```python
from build123d import *

# Parameters (mm, degrees)
SKETCH_1_R                         = 2.25
SM_BASE_FLANGE_1_DEPTH             = 5
FILLET_1_R                         = 30
SM_EDGE_FLANGE_1_STRIP_W           = 28
SM_EDGE_FLANGE_1_STRIP_H           = 5
SM_EDGE_FLANGE_1_STRIP_CUT_DEPTH   = 675
SM_EDGE_FLANGE_1_STRIP_2_W         = 28
SM_EDGE_FLANGE_1_STRIP_2_H         = 5
SM_EDGE_FLANGE_1_STRIP_CUT_2_DEPTH = 675
SM_EDGE_FLANGE_1_DEPTH             = 675
SM_EDGE_FLANGE_1_BEND_DEPTH        = 675
CUT_EXTRUDE_3_REACH                = 892.463
FILLET_2_R                         = 10
SKETCH_12_R                        = 5
CUT_EXTRUDE_4_DEPTH                = 891.463362525


# Sheet-metal steps are written as plain solids
with BuildPart() as part:
    # Sketch 1 → 基体-法兰1 (new body)
    with BuildSketch(Plane.XY):
        Polygon((0, 0), (0, 675), (45, 675), (45, 480), (165, 480), (165, 290), (535, 290), (535, 675), (580, 675), (580, 0), (523, 0), (523, 90), (57, 90), (57, 0), align=None)
        with Locations((154, 458)):
            Circle(SKETCH_1_R, mode=Mode.SUBTRACT)
        with Locations((45, 458)):
            Circle(SKETCH_1_R, mode=Mode.SUBTRACT)
        with Locations((154, 301)):
            Circle(SKETCH_1_R, mode=Mode.SUBTRACT)
        with Locations((45, 301)):
            Circle(SKETCH_1_R, mode=Mode.SUBTRACT)
        with BuildLine():
            Line((80, 133), (110, 133))
            ThreePointArc((110, 133), (150, 173), (110, 213))
            Line((110, 213), (80, 213))
            ThreePointArc((80, 213), (40, 173), (80, 133))
        make_face(mode=Mode.SUBTRACT)
    extrude(amount=-SM_BASE_FLANGE_1_DEPTH)

    # 圆角1
    fillet_1_edges = [part.edges().sort_by_distance(p)[0] for p in [
        (45, 480, -2.5),
        (165, 480, -2.5),
        (165, 290, -2.5),
        (535, 290, -2.5),
        (523, 90, -2.5),
        (57, 90, -2.5),
    ]]
    fillet(fillet_1_edges, radius=FILLET_1_R)

    # 边线-法兰1 strip (across the edge) → 边线-法兰1 strip cut (cut)
    with BuildSketch(Plane.XZ.offset(-675)):
        with Locations((-5, -2.5)):
            Rectangle(SM_EDGE_FLANGE_1_STRIP_W, SM_EDGE_FLANGE_1_STRIP_H)
    extrude(amount=SM_EDGE_FLANGE_1_STRIP_CUT_DEPTH, mode=Mode.SUBTRACT)

    # 边线-法兰1 strip 2 (across the edge) → 边线-法兰1 strip cut 2 (cut)
    with BuildSketch(Plane(origin=(580, 0, 0), x_dir=(-1, 0, 0), z_dir=(0, 1, 0))):
        with Locations((-5, -2.5)):
            Rectangle(SM_EDGE_FLANGE_1_STRIP_2_W, SM_EDGE_FLANGE_1_STRIP_2_H)
    extrude(amount=SM_EDGE_FLANGE_1_STRIP_CUT_2_DEPTH, mode=Mode.SUBTRACT)

    # 边线-法兰1 section (across the edge) → 边线-法兰1 (add)
    with BuildSketch(Plane.XZ.offset(-675)):
        with BuildLine():
            Line((0, 4), (0, 30))
            Line((0, 30), (5, 30))
            Line((5, 30), (5, 4))
            ThreePointArc((5, 4), (6.171572875, 1.171572875), (9, 0))
            Line((9, 0), (9, -5))
            ThreePointArc((9, -5), (2.636038969, -2.363961031), (0, 4))
        make_face()
    extrude(amount=SM_EDGE_FLANGE_1_DEPTH)

    # 边线-法兰1 section 2 (across the edge) → 边线-法兰1 bend (add)
    with BuildSketch(Plane(origin=(580, 0, 0), x_dir=(-1, 0, 0), z_dir=(0, 1, 0))):
        with BuildLine():
            Line((0, 4), (0, 30))
            Line((0, 30), (5, 30))
            Line((5, 30), (5, 4))
            ThreePointArc((5, 4), (6.171572875, 1.171572875), (9, 0))
            Line((9, 0), (9, -5))
            ThreePointArc((9, -5), (2.636038969, -2.363961031), (0, 4))
        make_face()
    extrude(amount=SM_EDGE_FLANGE_1_BEND_DEPTH)

    # 草图11 → 切除-拉伸3 (cut, up to next)
    with BuildSketch(Plane.XY, mode=Mode.PRIVATE) as cut_extrude_3_sk1:
        with BuildLine():
            Line((252.5, 110), (247.5, 110))
            ThreePointArc((247.5, 110), (241.5, 116), (247.5, 122))
            Line((247.5, 122), (252.5, 122))
            ThreePointArc((252.5, 122), (258.5, 116), (252.5, 110))
        make_face()
    cut_extrude_3_tool1 = extrude(cut_extrude_3_sk1.sketch, amount=-CUT_EXTRUDE_3_REACH, mode=Mode.PRIVATE) & part.part
    # 草图11 → 切除-拉伸3 (cut, up to next)
    with BuildSketch(Plane.XY, mode=Mode.PRIVATE) as cut_extrude_3_sk2:
        with BuildLine():
            Line((510.5, 110), (505.5, 110))
            ThreePointArc((505.5, 110), (499.5, 116), (505.5, 122))
            Line((505.5, 122), (510.5, 122))
            ThreePointArc((510.5, 122), (516.5, 116), (510.5, 110))
        make_face()
    cut_extrude_3_tool2 = extrude(cut_extrude_3_sk2.sketch, amount=-CUT_EXTRUDE_3_REACH, mode=Mode.PRIVATE) & part.part
    # 草图11 → 切除-拉伸3 (cut, up to next)
    with BuildSketch(Plane.XY, mode=Mode.PRIVATE) as cut_extrude_3_sk3:
        with BuildLine():
            Line((510.5, 224), (505.5, 224))
            ThreePointArc((505.5, 224), (499.5, 230), (505.5, 236))
            Line((505.5, 236), (510.5, 236))
            ThreePointArc((510.5, 236), (516.5, 230), (510.5, 224))
        make_face()
    cut_extrude_3_tool3 = extrude(cut_extrude_3_sk3.sketch, amount=-CUT_EXTRUDE_3_REACH, mode=Mode.PRIVATE) & part.part
    # 草图11 → 切除-拉伸3 (cut, up to next)
    with BuildSketch(Plane.XY, mode=Mode.PRIVATE) as cut_extrude_3_sk4:
        with BuildLine():
            Line((252.5, 224), (247.5, 224))
            ThreePointArc((247.5, 224), (241.5, 230), (247.5, 236))
            Line((247.5, 236), (252.5, 236))
            ThreePointArc((252.5, 236), (258.5, 230), (252.5, 224))
        make_face()
    cut_extrude_3_tool4 = extrude(cut_extrude_3_sk4.sketch, amount=-CUT_EXTRUDE_3_REACH, mode=Mode.PRIVATE) & part.part
    add(cut_extrude_3_tool1.solids().sort_by_distance((250, 116, 0))[0], mode=Mode.SUBTRACT)
    add(cut_extrude_3_tool2.solids().sort_by_distance((508, 116, 0))[0], mode=Mode.SUBTRACT)
    add(cut_extrude_3_tool3.solids().sort_by_distance((508, 230, 0))[0], mode=Mode.SUBTRACT)
    add(cut_extrude_3_tool4.solids().sort_by_distance((250, 230, 0))[0], mode=Mode.SUBTRACT)

    # 圆角2
    fillet_2_edges = [part.edges().sort_by_distance(p)[0] for p in [
        (2.5, 675, 30),
        (2.5, 0, 30),
        (577.5, 0, 30),
        (577.5, 675, 30),
    ]]
    fillet(fillet_2_edges, radius=FILLET_2_R)

    # 草图12 → 切除-拉伸4 (cut, through all)
    with BuildSketch(Plane(origin=(580, 0, 0), x_dir=(0, 0, -1), z_dir=(1, 0, 0))):
        with Locations((-15, 29)):
            Circle(SKETCH_12_R)
    extrude(amount=-CUT_EXTRUDE_4_DEPTH, mode=Mode.SUBTRACT)


solid = part.part
```
Model file for the job. Use its own axes, mm. A direction names the side the tool comes from. Coordinates: 2 decimals unless noted, no trailing zeros. Write each loop counter-clockwise with the first axis right and the second up, starting at its lowest first coordinate (ties: lowest second). Pieces come first, ordered by that corner, then holes. Notation, with made-up numbers: (41, 52) - (74, 52) arc R5 cw to (74, 58) - close; hole circle Ø2 at (28, -15.5). An arc over 180 degrees is marked (long way). One line per item, written item: value. Start each with the question number.
1. Probe line 1 (X direction, y = 275, z = 24); line 2 (Y direction, x = 576, z = 15); line 3 (Y direction, x = 154, z = -1.7). List the from-to ranges inside material, lowest first. Write a range as from..to.
2. Mould opens along X. For faces 6 (the flat face through (0, 342, 17)), 7 (the flat face through (22, 0, -1)), 8 (the cylindrical face through (525.979, 298.555, -2.535)) say: released by +X, released by -X, zero draft, split by the parting line, or undercut.
3. Slice it at C-C (x = 377.5). Write the cut outline in (y, z).
4. Slice it at A-A (y = 528.5). Write the cut outline in (x, z).
5. Tool access for faces 1 (the flat face through (18, 675, -1)), 2 (the cylindrical face through (40.01, 173.88, -2.46)), 3 (the cylindrical face through (65.555, 80.979, -2.535)), 4 (the flat face through (5, 342, 17)), 5 (the cylindrical face through (53.555, 489.021, -2.535)): list every direction of +Z, -Z, +X, -X, +Y, -Y with a clear straight run to the whole face (end or side of a thin tool).
6. Flat gauge pins, fed straight in: pin 1 (3.5 mm diameter, centred on x = 45, y = 458, fed in from +Z); pin 2 (1.5 mm diameter, centred on x = 101, z = -2.5, fed in from +Y); pin 3 (2.5 mm diameter, centred on y = 452, z = -2.5, fed in from -X); pin 4 (4 mm diameter, centred on y = 18, z = -2, fed in from +X). Where does each tip first touch, or does it go through?
7. Slice it at B-B (y = 333.5). Write the cut outline in (x, z).
Answers below:
1. line 1: x = 0..5, 575..580
1. line 2: y = 0..24, 34..675
1. line 3: y = 90..298.75, 303.25..455.75, 460.25..473.22
2. face 6: released by -X
2. face 7: zero draft
2. face 8: undercut
3. outline: (90, -5) - (290, -5) - (290, 0) - (90, 0) - close
4. outline: (0, 4) arc R9 ccw to (9, -5) - (45, -5) - (45, 0) - (9, 0) arc R4 cw to (5, 4) - (5, 30) - (0, 30) - close; (535, -5) - (571, -5) arc R9 ccw to (580, 4) - (580, 30) - (575, 30) - (575, 4) arc R4 cw to (571, 0) - (535, 0) - close
5. face 1: +Z, -Z, +X, -X, +Y
5. face 2: +Z, -Z
5. face 3: +Z, -Z, -Y
5. face 4: +Z, +Y, -Y
5. face 5: +Z, -Z, +Y
6. pin 1: passes through
6. pin 2: stops at y = 480
6. pin 3: stops at x = 1.69
6. pin 4: stops at x = 579.06
7. outline: (0, 4) arc R9 ccw to (9, -5) - (165, -5) - (165, 0) - (9, 0) arc R4 cw to (5, 4) - (5, 30) - (0, 30) - close; (535, -5) - (571, -5) arc R9 ccw to (580, 4) - (580, 30) - (575, 30) - (575, 4) arc R4 cw to (571, 0) - (535, 0) - close
